Print and shaded views of the part. All mm, measured from the part's lowest x, y and z. Give positions to 0.01 mm unless a question says otherwise; leave off trailing zeros. Loops run counter-clockwise (first coordinate to the right, second up) from the corner with the lowest first, then second, coordinate; pieces in that order, holes last. Notation, with made-up numbers: M -12.5,84.25 L 28.5,84.25 A23 cw 28.5,113.25 Z; hole C 5.5,42.25 d10. An arc over 180 degrees is marked long. Answer in a Markdown table with one row per item.
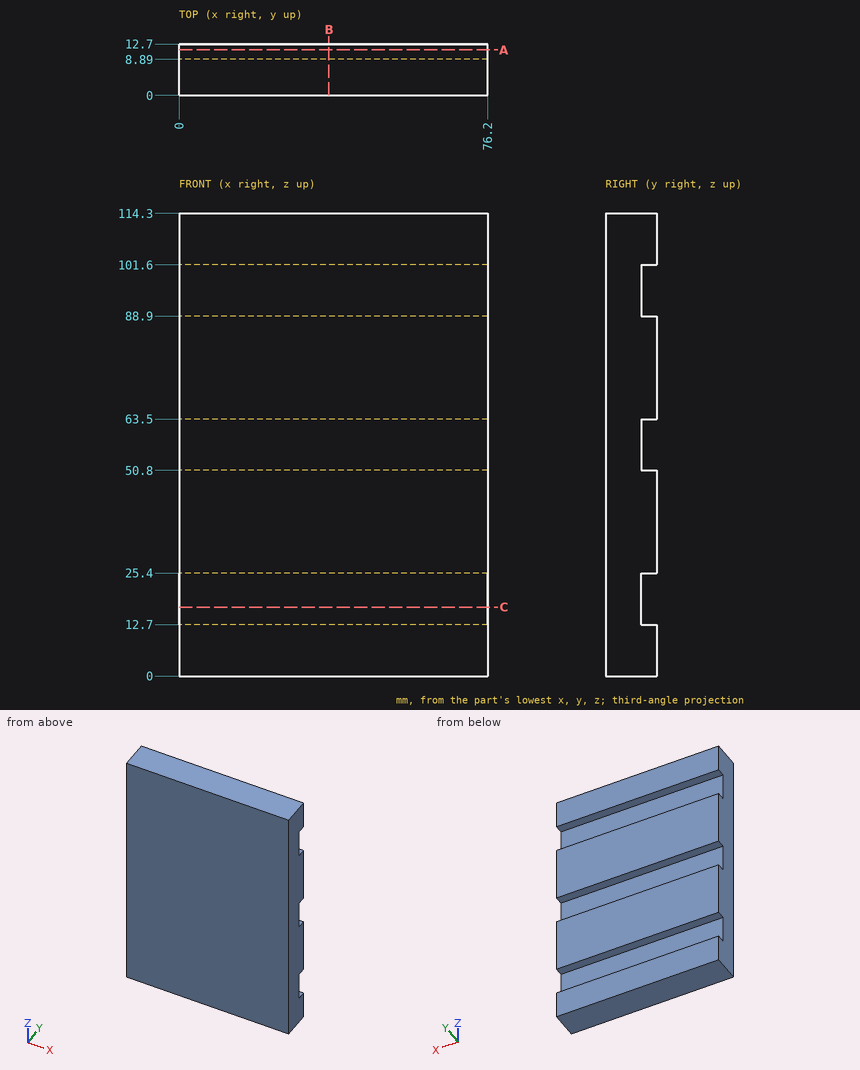
(1) Saw through at A-A, the plane y = 11.25. Give the cut face in (x, z).
Established:
| item | result |
|---|---|
| outline | M 0,0 L 76.2,0 L 76.2,12.7 L 0,12.7 Z; M 0,25.4 L 76.2,25.4 L 76.2,50.8 L 0,50.8 Z; M 0,63.5 L 76.2,63.5 L 76.2,88.9 L 0,88.9 Z; M 0,101.6 L 76.2,101.6 L 76.2,114.3 L 0,114.3 Z |
(2) Flat gauge pins, fed straight in: P1, Ø14, axis at x = 54, z = 17, coming from the +Y side; P2, Ø6.5, axis at x = 57, z = 97, coming from the +Y side. Where does each tip first touch, or does it go through?
Established:
| item | result |
|---|---|
| P1 | stops at y = 12.7 |
| P2 | stops at y = 8.89 |
(3) Wall check: L1, parallel to Z at x = 20.5, y = 10.75; L2, parallel to Y at x = 43, z = 98.5. Give the ranges that are in metal, low to high.
Established:
| item | result |
|---|---|
| L1 | z = 0 to 12.7, 25.4 to 50.8, 63.5 to 88.9, 101.6 to 114.3 |
| L2 | y = 0 to 8.89 |
(4) Saw through at C-C, the plane z = 17. Give the cut face in (x, y).
Established:
| item | result |
|---|---|
| outline | M 0,0 L 76.2,0 L 76.2,8.89 L 0,8.89 Z |
(5) Saw through at B-B, the plane x = 37. Give the cut face in (y, z), and give its area (3 significant figures).
Established:
| item | result |
|---|---|
| outline | M 0,0 L 12.7,0 L 12.7,12.7 L 8.89,12.7 L 8.89,25.4 L 12.7,25.4 L 12.7,50.8 L 8.89,50.8 L 8.89,63.5 L 12.7,63.5 L 12.7,88.9 L 8.89,88.9 L 8.89,101.6 L 12.7,101.6 L 12.7,114.3 L 0,114.3 Z |
| area | 1,310 mm2 |
